```python
from build123d import *

# Parameters (mm, degrees)
F1_DEPTH = 5.08
F4_DEPTH = 5.08


with BuildPart() as f1:
    # F0 (on Front) → F1 (new body)
    with BuildSketch(Plane.XZ):
        Polygon((47.7003678679, -8.732332848), (46.3905222714, -5.2393996157), (-41.3694269955, -5.2393996157), (-79.3550759554, 16.3731239736), (-81.8319656057, 12.019802605), (-41.3694269955, -8.732332848), align=None)
    extrude(amount=F1_DEPTH)


with BuildPart() as f4:
    # F3 (on Front) → F4 (new body)
    with BuildSketch(Plane.XZ):
        Polygon((44.6835160255, 1.7520437361), (44.6835160255, 6.6843586974), (-42.9144240916, 6.6843586974), (-71.3245719671, 21.2276466191), (-73.3251918619, 17.3194583635), (-42.9144240916, 1.7520437361), align=None)
    extrude(amount=F4_DEPTH)


solid = f4.part
```
Geometry check sheet. Reference: the model listing, model coordinates, mm. A direction names the side the tool comes from. Coordinates: 2 decimals unless noted, no trailing zeros. Order: outer loops, then holes, each group sorted by start corner. A loop starts at its lowest first (then second) coordinate and runs counter-clockwise, first axis right, second up.
Q1. Tool access check on faces 1 (the face through (1, -3, 6.684)), 2 (the face through (-72.31, -2.5, 19.3)). Record the directions out of +Z, -Z, +X, -X, +Y, -Y that give a thin tool (end or side, any length) a straight path to the whole face; none if there is none.
Reply:
face 1: +Z, +X, +Y, -Y
face 2: +Z, -X, +Y, -Y
Q2. Sectioned sample at B-B on x = -7. Record the cut outline in (y, z).
Reply:
outline: (-5.08, 1.75) - (0, 1.75) - (0, 6.68) - (-5.08, 6.68) - close
Q3. Sectioned sample at A-A on y = -3.85. Record the cut outline in (x, z).
Reply:
outline: (-73.33, 17.32) - (-42.91, 1.75) - (44.68, 1.75) - (44.68, 6.68) - (-42.91, 6.68) - (-71.32, 21.23) - close
Q4. Sectioned sample at C-C on z = 9.25. Record the cut outline in (x, y).
Reply:
outline: (-57.56, -5.08) - (-47.93, -5.08) - (-47.93, 0) - (-57.56, 0) - close
Q5. Thickness scan on probe 1 along Z at (x, y) = (-32, -0.65); probe 2 along X at (y, z) = (-3, 18.5); probe 3 along X at (y, z) = (-1.75, 15.5). Record the ranges inside material, lowest first.
Reply:
probe 1: z = 1.75 to 6.68
probe 2: x = -72.72 to -66
probe 3: x = -69.77 to -60.14
Q6. Depth check by flat-ended pin: pin 1 Ø1.5 at (x, y) = (2, -2.5) entering from +Z; pin 2 Ø2 at (y, z) = (-2, 11) entering from -X; pin 3 Ø1 at (y, z) = (-2.5, 15.5) entering from +X. Enter the tip coordinate at first touch or a pass-through.
Reply:
pin 1: stops at z = 6.68
pin 2: stops at x = -62.93
pin 3: stops at x = -59.16
